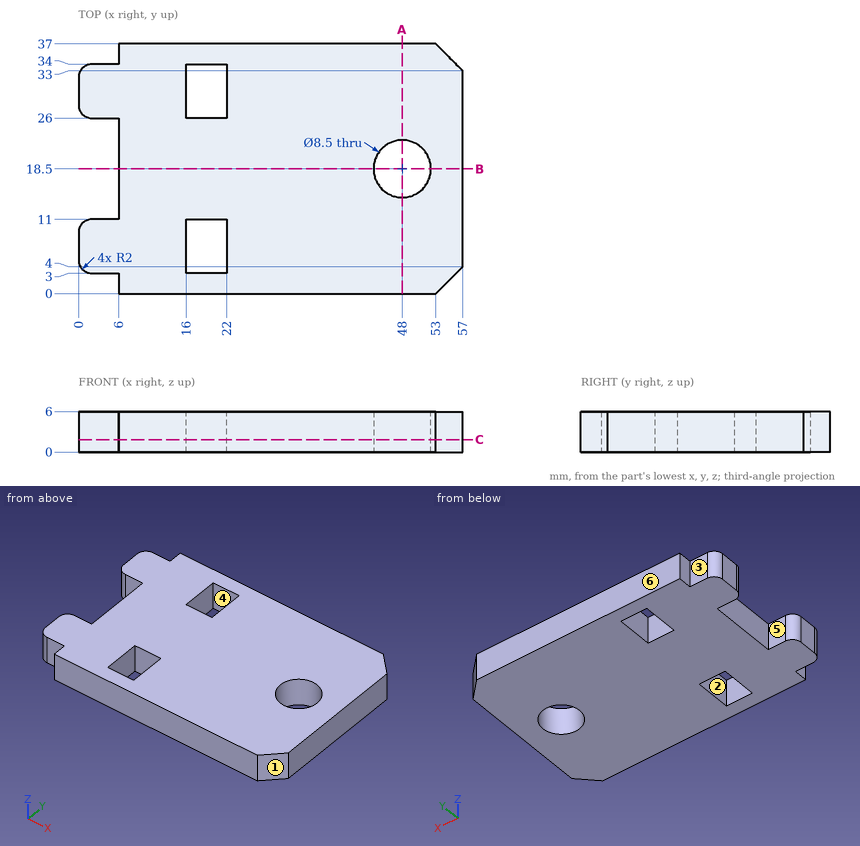
Can you work these out from the drawing? Everything is in mm from the part's minimum corner. A direction names the side the tool comes from. Give positions to 0.01 mm unless a question says otherwise; leave off trailing zeros. Order: outer loops, then holes, each group sorted by start corner. A loop starts at its lowest first (then second) coordinate and runs counter-clockwise, first axis right, second up.
Item 1: If we mould it in two halves opening along X, with no side actions, what happens to the marked faces 1, 2 and 3? For each: pulls with the +X half, pulls with the -X half, needs draft (parallel to the pull), parting line crosses it, or undercut.
Item 2: For the marked faces 4, 5 and 6, which set-ups out of +Z, -Z, +X, -X, +Y, -Y let a thin tool reach every point of the face, with its end or its side?
Item 3: I'm going to push flat-ended pins straight in: pin 1 (2.5 mm diameter, centred on y = 36, z = 3, fed in from -X); pin 2 (5 mm diameter, centred on x = 48, y = 18.5, fed in from +Z); pin 3 (3 mm diameter, centred on x = 3, z = 3.5, fed in from +Y). Where does each tip first touch, or does it pass through?
Item 4: I need wall thicknesses on line 1 (Y direction, x = 19, z = 3.85); line 2 (Y direction, x = 48, z = 2.75); line 3 (X direction, y = 30, z = 2.7). Which ranges of each line are inside material? Lowest first, please.
Item 5: If we section it at C-C, the plane z = 1.85: Write out the boundary of the cut face in (x, y), plus the area to 3 significant figures.
Item 6: If we section it at B-B, the plane y = 18.5: Write out the boundary of the cut face in (x, z).
Item 7: If we section it at A-A, the plane x = 48: Write out the boundary of the cut face in (y, z).
Values:
1. face 1: pulls with the +X half
1. face 2: undercut
1. face 3: needs draft
2. face 4: +Z, -Z
2. face 5: +Z, -Z, -X
2. face 6: +Z, -Z, +X, -X, +Y
3. pin 1: stops at x = 6
3. pin 2: passes through
3. pin 3: stops at y = 34
4. line 1: y = 0 to 3, 11 to 26, 34 to 37
4. line 2: y = 0 to 14.25, 22.75 to 37
4. line 3: x = 0 to 16, 22 to 57
5. outline: (0, 5) arc R2 ccw to (2, 3) - (6, 3) - (6, 0) - (53, 0) - (57, 4) - (57, 33) - (53, 37) - (6, 37) - (6, 34) - (2, 34) arc R2 ccw to (0, 32) - (0, 28) arc R2 ccw to (2, 26) - (6, 26) - (6, 11) - (2, 11) arc R2 ccw to (0, 9) - close; hole (16, 3) - (22, 3) - (22, 11) - (16, 11) - close; hole (16, 26) - (22, 26) - (22, 34) - (16, 34) - close; hole circle Ø8.5 at (48, 18.5)
5. area: 1,810 mm2
6. outline: (6, 0) - (43.75, 0) - (43.75, 6) - (6, 6) - close; (52.25, 0) - (57, 0) - (57, 6) - (52.25, 6) - close
7. outline: (0, 0) - (14.25, 0) - (14.25, 6) - (0, 6) - close; (22.75, 0) - (37, 0) - (37, 6) - (22.75, 6) - close
